Verification items for the finished model (mm, model axes). A direction names the side the tool comes from. Coordinates: 2 decimals unless noted, no trailing zeros. Write each loop counter-clockwise with the first axis right and the second up, starting at its lowest first coordinate (ties: lowest second). Pieces come first, ordered by that corner, then holes. Notation, with made-up numbers: M 55.5,-33 L 72.5,-33 A21 ccw 72.5,-16 Z; hole C 47,-2.5 d6. An arc over 180 degrees is marked long. Answer in a Markdown table with one row per item.
from build123d import *

# Parameters (mm, degrees)
SKETCH1_W           = 44
SKETCH1_H           = 20
BOSS_EXTRUDE1_DEPTH = 5
CUT_EXTRUDE1_REACH  = 50.59
SKETCH2_R           = 1.75
SKETCH3_R           = 2.5
CUT_EXTRUDE2_DEPTH  = 2
SKETCH4_W           = 10
SKETCH4_H           = 2.5
CUT_EXTRUDE3_DEPTH  = 2
FILLET1_R           = 1
FILLET2_R           = 0.5


with BuildPart() as part:
    # Sketch1 → Boss-Extrude1 (new body)
    with BuildSketch(Plane.XY):
        with Locations((22, 10)):
            Rectangle(SKETCH1_W, SKETCH1_H)
    extrude(amount=BOSS_EXTRUDE1_DEPTH)

    # Sketch2 → Cut-Extrude1 (cut, up to next)
    with BuildSketch(Plane.XY.offset(5), mode=Mode.PRIVATE) as cut_extrude1_sk1:
        with Locations((22, 15)):
            Circle(SKETCH2_R)
    cut_extrude1_tool1 = extrude(cut_extrude1_sk1.sketch, amount=-CUT_EXTRUDE1_REACH, mode=Mode.PRIVATE) & part.part
    # Sketch2 → Cut-Extrude1 (cut, up to next)
    with BuildSketch(Plane.XY.offset(5), mode=Mode.PRIVATE) as cut_extrude1_sk2:
        with Locations((22, 5)):
            Circle(SKETCH2_R)
    cut_extrude1_tool2 = extrude(cut_extrude1_sk2.sketch, amount=-CUT_EXTRUDE1_REACH, mode=Mode.PRIVATE) & part.part
    add(cut_extrude1_tool1.solids().sort_by_distance((22, 15, 5))[0], mode=Mode.SUBTRACT)
    add(cut_extrude1_tool2.solids().sort_by_distance((22, 5, 5))[0], mode=Mode.SUBTRACT)

    # Sketch3 → Cut-Extrude2 (cut)
    with BuildSketch(Plane.XY.offset(5)):
        with Locations((22, 15)):
            Circle(SKETCH3_R)
        with Locations((22, 5)):
            Circle(SKETCH3_R)
    extrude(amount=-CUT_EXTRUDE2_DEPTH, mode=Mode.SUBTRACT)

    # Sketch4 → Cut-Extrude3 (cut)
    with BuildSketch(Plane.XY.offset(5)):
        with Locations((10, 10)):
            Rectangle(SKETCH4_W, SKETCH4_H)
        Polygon((32.75, 5), (32.75, 8.75), (29, 8.75), (29, 11.25), (32.75, 11.25), (32.75, 15), (35.25, 15), (35.25, 11.25), (39, 11.25), (39, 8.75), (35.25, 8.75), (35.25, 5), align=None)
    extrude(amount=-CUT_EXTRUDE3_DEPTH, mode=Mode.SUBTRACT)

    # Fillet1
    fillet1_edges = [part.edges().sort_by_distance(p)[0] for p in [
        (44, 10, 5),
        (22, 20, 5),
        (0, 10, 5),
        (0, 20, 2.5),
        (44, 20, 2.5),
        (44, 0, 2.5),
        (0, 0, 2.5),
        (22, 0, 5),
    ]]
    fillet(fillet1_edges, radius=FILLET1_R)

    # Fillet2
    fillet2_edges = [part.edges().sort_by_distance(p)[0] for p in [
        (10, 11.25, 3),
        (15, 10, 3),
        (10, 8.75, 3),
        (5, 10, 3),
        (10, 11.25, 5),
        (5, 10, 5),
        (10, 8.75, 5),
        (15, 10, 5),
        (29, 10, 3),
        (29, 8.75, 4),
        (30.875, 11.25, 3),
        (29, 11.25, 4),
        (32.75, 13.125, 3),
        (32.75, 11.25, 4),
        (34, 15, 3),
        (32.75, 15, 4),
        (35.25, 13.125, 3),
        (35.25, 15, 4),
        (37.125, 11.25, 3),
        (39, 10, 3),
        (39, 11.25, 4),
        (37.125, 8.75, 3),
        (39, 8.75, 4),
        (35.25, 6.875, 3),
        (34, 5, 3),
        (35.25, 5, 4),
        (32.75, 6.875, 3),
        (32.75, 5, 4),
        (30.875, 8.75, 3),
        (29, 10, 5),
        (30.875, 8.75, 5),
        (32.75, 6.875, 5),
        (34, 5, 5),
        (35.25, 6.875, 5),
        (37.125, 8.75, 5),
        (39, 10, 5),
        (37.125, 11.25, 5),
        (35.25, 13.125, 5),
        (34, 15, 5),
        (32.75, 13.125, 5),
        (30.875, 11.25, 5),
    ]]
    fillet(fillet2_edges, radius=FILLET2_R)


solid = part.part
1) Sectioned sample at B-B (z = 1.6). Record the cut outline in (x, y), then the cut area to 3 significant figures.
Response values:
| item | result |
|---|---|
| outline | M 0,1 A1 ccw 1,0 L 43,0 A1 ccw 44,1 L 44,19 A1 ccw 43,20 L 1,20 A1 ccw 0,19 Z; hole C 22,5 d3.5; hole C 22,15 d3.5 |
| area | 860 mm² |
2) Depth check by flat-ended pin: pin 1 (4 mm diameter, centred on x = 22, y = 5, fed in from +Z). Enter the tip coordinate at first touch or a pass-through.
Response values:
| item | result |
|---|---|
| pin 1 | stops at z = 3 |
3) Release check for a two-part mould opening along Y. For faces 3 (the face through (0.285, 19.699, 2.028)), 4 (the face through (32.75, 7, 4)), 5 (the face through (43.699, 0.285, 2.028)) record: +Y half, -Y half, draft (parallel to the pull), parting line (faces both ways), or undercut.
Response values:
| item | result |
|---|---|
| face 3 | +Y half |
| face 4 | undercut |
| face 5 | -Y half |
4) Tool access check on faces 1 (the face through (22, 20, 2)), 2 (the face through (39, 10, 4)). Record the directions out of +Z, -Z, +X, -X, +Y, -Y that give a thin tool (end or side, any length) a straight path to the whole face; none if there is none.
Response values:
| item | result |
|---|---|
| face 1 | +Z, -Z, +X, -X, +Y |
| face 2 | +Z |
5) Thickness scan on L1, parallel to Y at x = 22, z = 1.1; L2, parallel to Y at x = 22, z = 3.7; L3, parallel to X at y = 9.75, z = 3.85. Record the ranges inside material, lowest first. Write a range as [from, to].
Response values:
| item | result |
|---|---|
| L1 | y = [0, 3.25], [6.75, 13.25], [16.75, 20] |
| L2 | y = [0, 2.5], [7.5, 12.5], [17.5, 20] |
| L3 | x = [0, 5], [15, 29], [39, 44] |
6) Sectioned sample at A-A (x = 22). Record the cut outline in (y, z), then the cut area to 3 significant figures.
Response values:
| item | result |
|---|---|
| outline | M 0,0 L 3.25,0 L 3.25,3 L 2.5,3 L 2.5,5 L 1,5 A1 ccw 0,4 Z; M 6.75,0 L 13.25,0 L 13.25,3 L 12.5,3 L 12.5,5 L 7.5,5 L 7.5,3 L 6.75,3 Z; M 16.75,0 L 20,0 L 20,4 A1 ccw 19,5 L 17.5,5 L 17.5,3 L 16.75,3 Z |
| area | 58.6 mm² |
